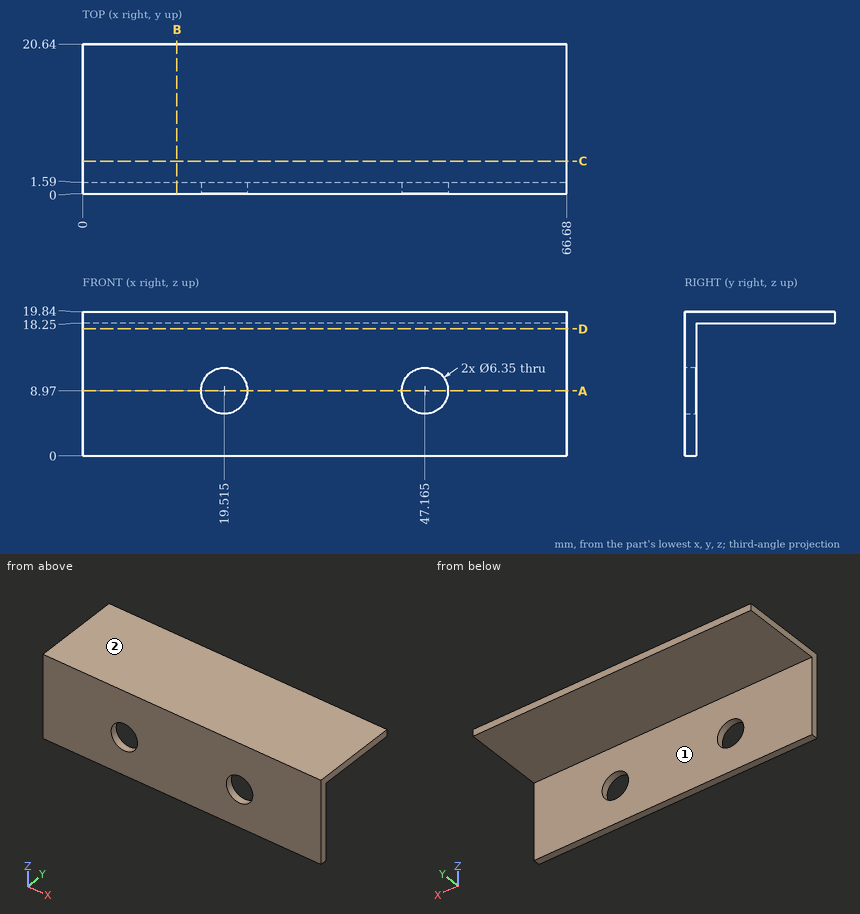
Geometry check sheet. Reference: drawing and pictorial views, mm from the part's lowest x, y, z. A direction names the side the tool comes from. Give positions to 0.01 mm unless a question says otherwise; leave off trailing zeros. Order: outer loops, then holes, each group sorted by start corner. A loop starts at its lowest first (then second) coordinate and runs counter-clockwise, first axis right, second up. Notation, with made-up numbers: (55, 75) -> (72, 75) arc R24 ccw to (72, 109) -> close; hole circle Ø7 at (66.5, 85). An arc over 180 degrees is marked (long way). Use CSV: the item, a comma, the result in double quotes. Start each with the question number.
1) Material ranges on line 1 (X direction, y = 1.1, z = 8.97); line 2 (Z direction, x = 4.5, y = 11); line 3 (Y direction, x = 19, z = 5.25), recorded low to high. Write a range as from..to.
2) Set-up check for the marked faces 1 and 2: record each of +Z, -Z, +X, -X, +Y, -Y from which the full face is reachable in a straight line by a thin tool's end or side.
3) Sectioned sample at A-A, the plane z = 8.97. Record the boundary of the cut face in (x, y).
4) Sectioned sample at B-B, the plane x = 13. Record the boundary of the cut face in (y, z), plus the area to 3 significant figures.
5) Go/stop test with flat-tipped pins: P1, Ø5.5, axis at x = 34.5, y = 11, coming from the -Z side; P2, Ø5, axis at x = 47.165, z = 8.97, coming from the -Y side; P3, Ø7.5, axis at x = 19.515, z = 8.97, coming from the +Y side; P4, Ø5, axis at y = 13.5, z = 16, coming from the -X side. Record where each tip stops, or that it passes through.
6) Sectioned sample at C-C, the plane y = 4.5. Record the boundary of the cut face in (x, z).
7) Sectioned sample at D-D, the plane z = 17.5. Record the boundary of the cut face in (x, y), plus the area to 3 significant figures.
Recorded:
1,line 1,"0..16.34, 22.69..43.99, 50.34..66.68"
1,line 2,"18.25..19.84"
1,line 3,"0..1.59"
2,face 1,"-Z, +X, -X, +Y"
2,face 2,"+Z, +X, -X, +Y, -Y"
3,outline,"(0, 0) -> (16.34, 0) -> (16.34, 1.59) -> (0, 1.59) -> close; (22.69, 0) -> (43.99, 0) -> (43.99, 1.59) -> (22.69, 1.59) -> close; (50.34, 0) -> (66.68, 0) -> (66.68, 1.59) -> (50.34, 1.59) -> close"
4,outline,"(0, 0) -> (1.59, 0) -> (1.59, 18.25) -> (20.64, 18.25) -> (20.64, 19.84) -> (0, 19.84) -> close"
4,area,"61.8 mm2"
5,P1,"z = 18.25"
5,P2,"through"
5,P3,"y = 1.59"
5,P4,"x = 0"
6,outline,"(0, 18.25) -> (66.68, 18.25) -> (66.68, 19.84) -> (0, 19.84) -> close"
7,outline,"(0, 0) -> (66.68, 0) -> (66.68, 1.59) -> (0, 1.59) -> close"
7,area,"106 mm2"
